Work out the finished part from the listing and answer in its coordinate system (mm). A direction names the side the tool comes from. Round coordinates to 2 decimals unless told otherwise and drop trailing zeros. Write each loop counter-clockwise with the first axis right and the second up, starting at its lowest first coordinate (ties: lowest second). Pieces come first, ordered by that corner, then holes.
Autodesk Inventor part; units mm, degrees
ref_plane "YZ Plane" through (0, 0, 0) normal (1, 0, 0) x (0, 1, 0)
ref_plane "XZ Plane" through (0, 0, 0) normal (0, 1, 0) x (-1, 0, 0)
ref_plane "XY Plane" through (0, 0, 0) normal (0, 0, 1) x (1, 0, 0)
sketch "Эскиз1" plane through (0, 0, 0) normal (0, 1, 0) x (-1, 0, 0)
  circle A0 centre (0, 0) radius 12.5
  circle A1 centre (0, 0) radius 15
  dimension "d0" = 25
  dimension "d1" = 30
extrude "Выдавливание1" add sketch "Эскиз1" along normal blind 31
sketch "Эскиз2" plane through (0, 0, 0) normal (0, -1, 0) x (1, 0, 0)
  line L0 (0, 20) -> (0, -20)
  circle A0 centre (0, 20) radius 2
  circle A1 centre (0, -20) radius 2
  circle A2 centre (0, 20) radius 3
  circle A3 centre (0, -20) radius 3
  line L1 (15, 10) -> (15, -10)
  circle A4 centre (0, 0) radius 15
  line L2 (-15, 10) -> (-15, -10)
  line L3 (3, 20) -> (15, 10)
  line L4 (15, -10) -> (3, -20)
  line L5 (-15, -10) -> (-3, -20)
  line L6 (-3, 20) -> (-15, 10)
  point P0 (15, 0)
  point P1 (-15, 0)
  dimension "d4" = 40
  dimension "d5" = 4
  dimension "d6" = 4
  dimension "d7" = 6
  dimension "d8" = 6
  dimension "d9" = 20
  dimension "d10" = 20
  dimension "d11" = 10
  dimension "d12" = 10
extrude "Выдавливание2" add sketch "Эскиз2" against normal blind 8 contours A2 | A2 L3 L1 A4 L0 | L0 A4 L2 L6 A2 | A4 L1 L4 A3 L0 | L0 A3 L5 L2 A4 | A3
fillet "Сопряжение1" radius 10 4 edges at (-15, 4, 10) (-15, 4, -10) (15, 4, 10) (15, 4, -10)
fillet "Сопряжение2" radius 10 4 edges at (3, 4, 20) (-3, 4, 20) (3, 4, -20) (-3, 4, -20)
properties part number "conder"
Q1. Find section A-A (x = 0). Determine the outline of the cut face in (y, z).
Q2. The mould has two halves that part along X. Classify faces 3 (the face through (-11.923, 15.283, -3.755)), 4 (the face through (15, 4, 0)), 5 (the face through (-14.03, 4.06, -9.61)): +X half, -X half, draft (parallel to the pull), parting line (faces both ways), or undercut.
Q3. A tool of negligible diameter and unlimited length cuts with its end or side. For faces 1 (the face through (-3.8, 4.1, -19.6)), 2 (the face through (0, 8, 16)), from which of +Z, -Z, +X, -X, +Y, -Y can it reach the whole face along a straight path? Write none if from no direction.
Q4. Find section B-B (x = 6.5). Determine the outline of the cut face in (y, z), plus the area to 3 significant figures.
Q5. Find section D-D (y = 10). Determine the outline of the cut face in (x, z).
Q6. Find the intervals of material crossed by L1, parallel to Y at x = -6, z = -14; L2, parallel to X at y = 4.5, z = -20; L3, parallel to X at y = 13, z = -6.5, in increasing order.
Q7. Given pin 1 (6 mm diameter, centred on x = 1, y = 18, fed in from +Z); pin 2 (1 mm diameter, centred on x = 3, y = 6, fed in from -Z); pin 3 (2 mm diameter, centred on y = 3, z = -11, fed in from +X), each flat-ended and moving along its own axis, determine where each tip first touches the part or whether it passes through.
Q8. Find section C-C (z = 2.5). Determine the outline of the cut face in (x, y).
Report:
1. outline: (0, -23) - (8, -23) - (8, -22) - (0, -22) - close; (0, -18) - (8, -18) - (8, -15) - (31, -15) - (31, -12.5) - (0, -12.5) - close; (0, 12.5) - (31, 12.5) - (31, 15) - (8, 15) - (8, 18) - (0, 18) - close; (0, 22) - (8, 22) - (8, 23) - (0, 23) - close
2. face 3: undercut
2. face 4: +X half
2. face 5: -X half
3. face 1: -Z, -X, +Y, -Y
3. face 2: +Z, +Y
4. outline: (0, -17.08) - (8, -17.08) - (8, -13.52) - (31, -13.52) - (31, -10.68) - (0, -10.68) - close; (0, 10.68) - (31, 10.68) - (31, 13.52) - (8, 13.52) - (8, 17.08) - (0, 17.08) - close
4. area: 233 mm2
5. outline: circle Ø30 at (0, 0); hole circle Ø25 at (0, 0)
6. L1: y = 0 to 8
6. L2: x = -3.5 to -2, 2 to 3.5
6. L3: x = -13.52 to -10.68, 10.68 to 13.52
7. pin 1: stops at z = 15
7. pin 2: stops at z = -21.66
7. pin 3: stops at x = 13.84
8. outline: (-15, 0) - (-12.25, 0) - (-12.25, 31) - (-14.79, 31) - (-14.79, 8) - (-15, 8) - close; (12.25, 0) - (15, 0) - (15, 8) - (14.79, 8) - (14.79, 31) - (12.25, 31) - close
